Read the model definition and answer for the solid it produces. Units are mm, in the model's axes. A direction names the side the tool comes from. Coordinates: 2 decimals unless noted, no trailing zeros. Order: outer loops, then holes, each group sorted by start corner. A loop starts at its lowest first (then second) coordinate and runs counter-clockwise, first axis right, second up. Notation, with made-up numbers: (56, 62.25) - (97, 62.25) arc R7 ccw to (97, 73.25) - close; hole circle Ø6 at (-33, 24). An arc over 180 degrees is marked (long way). Answer as a JSON object with one key per item and string values. Group by question number.
Autodesk Inventor part; units mm, degrees
ref_plane "YZ Plane" through (0, 0, 0) normal (1, 0, 0) x (0, 1, 0)
ref_plane "XZ Plane" through (0, 0, 0) normal (0, 1, 0) x (-1, 0, 0)
ref_plane "XY Plane" through (0, 0, 0) normal (0, 0, 1) x (1, 0, 0)
sketch "スケッチ1" plane through (0, 0, 0) normal (0, 1, 0) x (-1, 0, 0)
  circle A0 centre (0, 0) radius 3
  dimension "d0" = 6
extrude "押し出し1" add sketch "スケッチ1" along normal mid plane 60
sketch "スケッチ2" plane through (0, 30, 0) normal (0, 1, 0) x (1, 0, 0)
  point P0 (0, 0)
  point P1 (0, 0)
hole "穴1" at (0, 30, 0) direction (0, -1, 0) diameter 2.459 depth 10 countersink diameter 3.4 countersink angle 90
sketch "スケッチ3" plane through (0, -30, 0) normal (0, -1, 0) x (1, 0, 0)
  point P0 (0, 0)
  point P1 (0, 0)
hole "穴2" at (0, -30, 0) direction (0, 1, 0) diameter 2.459 depth 10 countersink diameter 3.4 countersink angle 90
chamfer "面取り1" distance 0.25 angle 45 2 edges at (3, -30, 0) (3, 30, 0)
properties part number "Spacer_M3D6L60" material "アルミニウム 6061"
1. A cutting plane is placed at A-A on x = 0. Write down the section's boundary in (y, z), and give its area (3 significant figures).
2. Straight lines are drawn through the part: L1, parallel to Z at x = 0, y = 25.5; L2, parallel to Y at x = -1.1, z = -0.25; L3, parallel to Z at x = 1.85, y = 1. For each, find the intervals that lie inside material, in ascending order.
3. A cutting plane is placed at B-B on z = 0. Write down the section's boundary in (x, y).
4. A cutting plane is placed at C-C on y = 11.5. Write down the section's boundary in (x, z), and give its area (3 significant figures).
5. For faces 1 (the flat face through (-2, -30, 0)), 2 (the cylindrical face through (0.748, -24.698, 0.976)), 3 (the flat face through (0, 20, 0)), determine the directions among +Z, -Z, +X, -X, +Y, -Y from which every point of the face is accessible in a straight line to the end or side of a thin tool.
6. Given pin 1 (0.7 mm diameter, centred on x = 0.5, z = -0.5, fed in from +Y); pin 2 (2 mm diameter, centred on x = 0, z = 0, fed in from -Y), each flat-ended and moving along its own axis, determine where each tip first touches the part or whether it passes through.
7. A cutting plane is placed at D-D on y = 22.5. Write down the section's boundary in (x, z).
8. For a pull along X with two mould halves and no side action, classify faces 4 (the flat face through (-2, 30, 0)), 5 (the cylindrical face through (3, 0, 0)), 6 (the cylindrical face through (0.748, 24.698, -0.976)) as pulls with the +X half, pulls with the -X half, needs draft (parallel to the pull), parting line crosses it, or undercut.
Derived:
{
 "1": {"outline": "(-30, -2.75) - (-29.75, -3) - (29.75, -3) - (30, -2.75) - (30, -1.7) - (29.53, -1.23) - (20, -1.23) - (20, 1.23) - (29.53, 1.23) - (30, 1.7) - (30, 2.75) - (29.75, 3) - (-29.75, 3) - (-30, 2.75) - (-30, 1.7) - (-29.53, 1.23) - (-20, 1.23) - (-20, -1.23) - (-29.53, -1.23) - (-30, -1.7) - close", "area": "310 mm2"},
 "2": {"L1": "z = -3 to -1.23, 1.23 to 3", "L2": "y = -20 to 20", "L3": "z = -2.36 to 2.36"},
 "3": {"outline": "(-3, -29.75) - (-2.75, -30) - (-1.7, -30) - (-1.23, -29.53) - (-1.23, -20) - (1.23, -20) - (1.23, -29.53) - (1.7, -30) - (2.75, -30) - (3, -29.75) - (3, 29.75) - (2.75, 30) - (1.7, 30) - (1.23, 29.53) - (1.23, 20) - (-1.23, 20) - (-1.23, 29.53) - (-1.7, 30) - (-2.75, 30) - (-3, 29.75) - close"},
 "4": {"outline": "circle Ø6 at (0, 0)", "area": "28.3 mm2"},
 "5": {"face 1": "+Z, -Z, +X, -X, -Y", "face 2": "-Y", "face 3": "+Y"},
 "6": {"pin 1": "stops at y = 20", "pin 2": "stops at y = -20"},
 "7": {"outline": "circle Ø6 at (0, 0); hole circle Ø2.46 at (0, 0)"},
 "8": {"face 4": "needs draft", "face 5": "parting line crosses it", "face 6": "undercut"}
}
